The listing builds one solid part. Answer for the finished solid, in the listing's coordinates (mm). A direction names the side the tool comes from. Give positions to 0.01 mm unless a question says otherwise; leave off trailing zeros. Write each loop counter-clockwise with the first axis right and the second up, starting at its lowest first coordinate (ties: lowest second). Pieces come first, ordered by that corner, then holes. Notation, with made-up numbers: (88.5, 17) - (93.5, 17) arc R16 ccw to (93.5, 35) - close; hole circle Ø2 at (-1.5, 74.5). An arc over 180 degrees is marked (long way). Return JSON: item names as keys, results as strings.
from build123d import *

# Parameters (mm, degrees)
SKETCH1_W           = 154
SKETCH1_H           = 116
BOSS_EXTRUDE1_DEPTH = 5
SKETCH2_W           = 150
SKETCH2_H           = 102
CUT_EXTRUDE1_DEPTH  = 3
SKETCH3_R           = 1.5
CUT_EXTRUDE2_DEPTH  = 97.529788149
FILLET1_R           = 3
FILLET2_R           = 3
FILLET3_R           = 3
FILLET4_R           = 3


with BuildPart() as part:
    # Sketch1 → Boss-Extrude1 (new body)
    with BuildSketch(Plane(origin=(0, 0, 0), x_dir=(1, 0, 0), z_dir=(0, 1, 0))):
        Rectangle(SKETCH1_W, SKETCH1_H)
    extrude(amount=BOSS_EXTRUDE1_DEPTH)

    # Sketch2 → Cut-Extrude1 (cut)
    with BuildSketch(Plane(origin=(0, 5, 0), x_dir=(1, 0, 0), z_dir=(0, 1, 0))):
        Rectangle(SKETCH2_W, SKETCH2_H)
    extrude(amount=-CUT_EXTRUDE1_DEPTH, mode=Mode.SUBTRACT)

    # Sketch3 → Cut-Extrude2 (cut, through all)
    with BuildSketch(Plane(origin=(0, 5, 0), x_dir=(1, 0, 0), z_dir=(0, 1, 0))):
        with Locations(Location((-73.5, 54.5, 0), (0, 0, 270))):
            Circle(SKETCH3_R)
        with Locations(Location((73.5, 54.5, 0), (0, 0, 270))):
            Circle(SKETCH3_R)
        with Locations(Location((73.5, -54.5, 0), (0, 0, 270))):
            Circle(SKETCH3_R)
        with Locations(Location((-73.5, -54.5, 0), (0, 0, 270))):
            Circle(SKETCH3_R)
    extrude(amount=-CUT_EXTRUDE2_DEPTH, mode=Mode.SUBTRACT)

    # Fillet1
    fillet1_edges = [part.edges().sort_by_distance(p)[0] for p in [
        (77, 2.5, 58),
    ]]
    fillet(fillet1_edges, radius=FILLET1_R)

    # Fillet2
    fillet2_edges = [part.edges().sort_by_distance(p)[0] for p in [
        (-77, 2.5, 58),
    ]]
    fillet(fillet2_edges, radius=FILLET2_R)

    # Fillet3
    fillet3_edges = [part.edges().sort_by_distance(p)[0] for p in [
        (-77, 2.5, -58),
    ]]
    fillet(fillet3_edges, radius=FILLET3_R)

    # Fillet4
    fillet4_edges = [part.edges().sort_by_distance(p)[0] for p in [
        (77, 2.5, -58),
    ]]
    fillet(fillet4_edges, radius=FILLET4_R)


solid = part.part
Item 1: A cutting plane is placed at C-C on x = 19. Determine the outline of the cut face in (y, z).
Answer below:
{"outline": "(0, -58) - (5, -58) - (5, -51) - (2, -51) - (2, 51) - (5, 51) - (5, 58) - (0, 58) - close"}
Item 2: A cutting plane is placed at B-B on z = -20. Determine the outline of the cut face in (x, y).
Answer below:
{"outline": "(-77, 0) - (77, 0) - (77, 5) - (75, 5) - (75, 2) - (-75, 2) - (-75, 5) - (-77, 5) - close"}
Item 3: For faces 5 (the face through (75, 4, 1)), 6 (the face through (0, 5, -52)), determine the directions among +Z, -Z, +X, -X, +Y, -Y from which every point of the face is accessible in a straight line to the end or side of a thin tool.
Answer below:
{"face 5": "+Y", "face 6": "+Z, -Z, +X, -X, +Y"}
Item 4: Flat-ended cylindrical pins translate along their axes: P1, Ø5, axis at x = -73.5, z = -54.5, coming from the +Y side; P2, Ø6, axis at x = 30.5, z = 44.5, coming from the +Y side. Find the tip coordinate at first contact, or state that the pin passes through.
Answer below:
{"P1": "stops at y = 5", "P2": "stops at y = 2"}
Item 5: The mould has two halves that part along X. Classify faces 1 (the face through (-76.14, 2.54, -57.1)), 2 (the face through (-1, 0, -1)), 3 (the face through (77, 2, 1)), 4 (the face through (-75, 4, 1)): +X half, -X half, draft (parallel to the pull), parting line (faces both ways), or undercut.
Answer below:
{"face 1": "-X half", "face 2": "draft", "face 3": "+X half", "face 4": "undercut"}
Item 6: A cutting plane is placed at A-A on y = 3.75. Determine the outline of the cut face in (x, z), then the cut area to 3 significant figures.
Answer below:
{"outline": "(-77, -55) arc R3 ccw to (-74, -58) - (74, -58) arc R3 ccw to (77, -55) - (77, 55) arc R3 ccw to (74, 58) - (-74, 58) arc R3 ccw to (-77, 55) - close; hole circle Ø3 at (-73.5, -54.5); hole (-75, -51) - (75, -51) - (75, 51) - (-75, 51) - close; hole circle Ø3 at (-73.5, 54.5); hole circle Ø3 at (73.5, -54.5); hole circle Ø3 at (73.5, 54.5)", "area": "2,530 mm²"}
Item 7: Consider L1, parallel to Z at x = -73.5, y = 2.1; L2, parallel to X at y = 3.9, z = -54.5; L3, parallel to X at y = 3.4, z = -47.5. Determine where each line is inside the solid, lowest interval first.
Answer below:
{"L1": "z = -58 to -56, -53 to -51, 51 to 53, 56 to 58", "L2": "x = -77 to -75, -72 to 72, 75 to 77", "L3": "x = -77 to -75, 75 to 77"}
